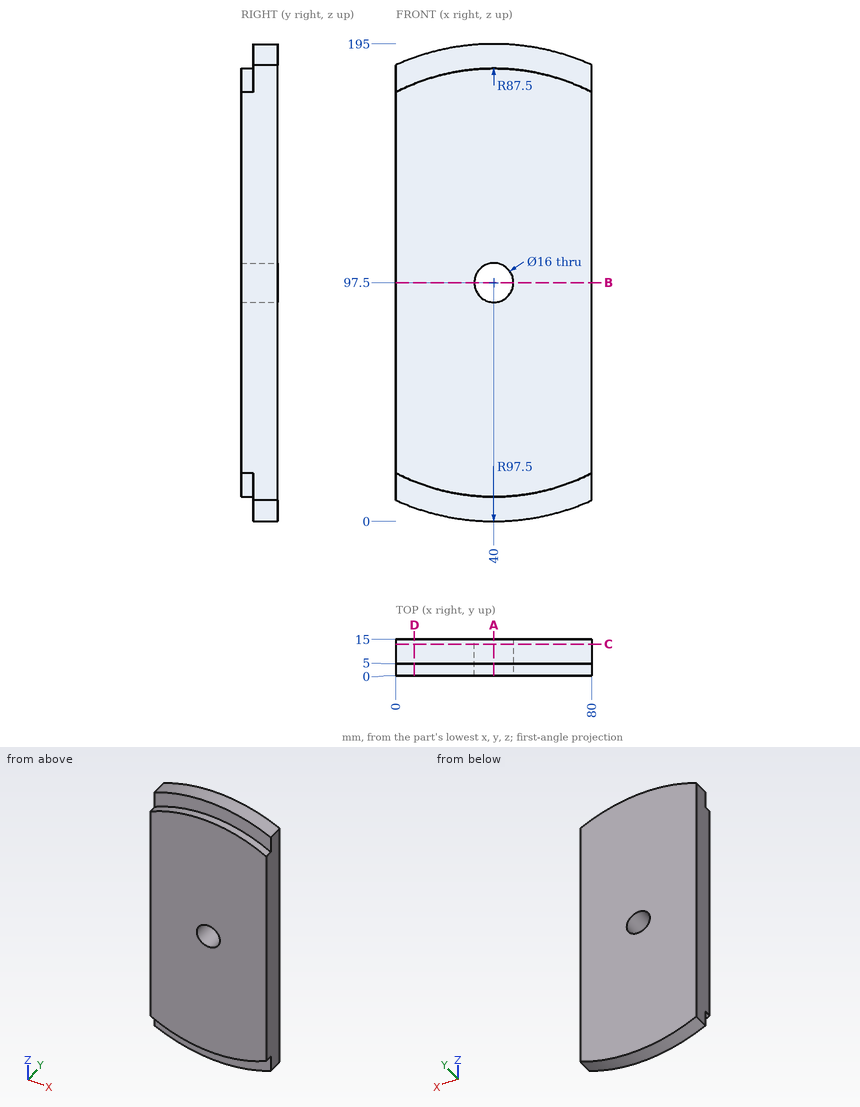
Geometry check sheet. Reference: drawing and pictorial views, mm from the part's lowest x, y, z. Coordinates: 2 decimals unless noted, no trailing zeros. Order: outer loops, then holes, each group sorted by start corner. A loop starts at its lowest first (then second) coordinate and runs counter-clockwise, first axis right, second up. Notation, with made-up numbers: (21.5, 55) -> (36.5, 55) arc R34 cw to (36.5, 90) -> close; hole circle Ø11 at (22, 61.25). An arc over 180 degrees is marked (long way). Write item = value, one per line. Start each with the question number.
1) Cross-section at C-C (y = 13). Enter the section's corners in (x, z), then the cut area to 3 significant figures.
2) Go/stop test with flat-tipped pins: P1, Ø6, axis at x = 38.5, z = 12, coming from the -Y side; P2, Ø4, axis at x = 10, y = 7.5, coming from the -Z side; P3, Ø6, axis at x = 17, y = 2.5, coming from the -Z side; P4, Ø6, axis at x = 30.5, z = 188.5, coming from the -Y side. Record where each tip stops, or that it passes through.
3) Cross-section at B-B (z = 97.5). Enter the section's corners in (x, y).
4) Material ranges on L1, parallel to Z at x = 40, y = 3.75; L2, parallel to Z at x = 40, y = 7.5; L3, parallel to Y at x = 13, z = 10, recorded low to high.
5) Cross-section at A-A (x = 40). Enter the section's corners in (y, z).
6) Cross-section at D-D (x = 7.5). Enter the section's corners in (y, z).
Ans:
q1.outline = (0, 8.58) arc R97.5 ccw to (80, 8.58) -> (80, 186.42) arc R97.5 ccw to (0, 186.42) -> close; hole circle Ø16 at (40, 97.5)
q1.area = 14,900 mm²
q2.P1 = 0
q2.P2 = 4.11
q2.P3 = 2.36
q2.P4 = 5
q3.outline = (0, 0) -> (32, 0) -> (32, 15) -> (0, 15) -> close; (48, 0) -> (80, 0) -> (80, 15) -> (48, 15) -> close
q4.L1 = 10 to 89.5, 105.5 to 185
q4.L2 = 0 to 89.5, 105.5 to 195
q4.L3 = 5 to 15
q5.outline = (0, 10) -> (5, 10) -> (5, 0) -> (15, 0) -> (15, 89.5) -> (0, 89.5) -> close; (0, 105.5) -> (15, 105.5) -> (15, 195) -> (5, 195) -> (5, 185) -> (0, 185) -> close
q6.outline = (0, 16.26) -> (5, 16.26) -> (5, 5.58) -> (15, 5.58) -> (15, 189.42) -> (5, 189.42) -> (5, 178.74) -> (0, 178.74) -> close
